Could you check a few things on this model? Use its own coordinates, in mm. Face numbers are marked on the shaded views. A direction names the side the tool comes from. Give positions to 0.01 mm unless a question says otherwise; leave off trailing zeros. Order: outer loops, then holes, each group sorted by start corner. A loop starts at its lowest first (then second) coordinate and runs counter-clockwise, first axis right, second up. Notation, with made-up numbers: M 63.5,68 L 77.5,68 A33 ccw 77.5,102 Z; hole C -13,-21 d2. An arc over 180 degrees is marked long. Answer in a Markdown table with one row per item. Add a question column.
```python
from build123d import *

# Parameters (mm, degrees)
SKETCH_2_R      = 65
SKETCH_2_R_2    = 37.5
EXTRUDE_1_DEPTH = 10
EXTRUDE_2_DEPTH = 50
CHAMFER_1_SIZE  = 10
FILLET_2_R      = 1


with BuildPart() as part:
    # 草圖2 → 填料-伸長1 (new body)
    with BuildSketch(Plane(origin=(0, 0, 0), x_dir=(1, 0, 0), z_dir=(0, 1, 0))):
        with Locations(Location((0, 0, 0), (0, 0, 270))):
            Circle(SKETCH_2_R)
        with Locations(Location((0, 0, 0), (0, 0, 270))):
            Circle(SKETCH_2_R_2, mode=Mode.SUBTRACT)
    extrude(amount=EXTRUDE_1_DEPTH)

    # 草圖3 → 填料-伸長2 (add)
    with BuildSketch(Plane(origin=(0, 10, 0), x_dir=(1, 0, 0), z_dir=(0, 1, 0))):
        with BuildLine():
            Line((-32.475952642, -18.75), (-41.13620668, -23.75))
            ThreePointArc((-41.13620668, -23.75), (0, 47.5), (41.13620668, -23.75))
            Line((41.13620668, -23.75), (32.475952642, -18.75))
            ThreePointArc((32.475952642, -18.75), (0, 37.5), (-32.475952642, -18.75))
        make_face()
    extrude(amount=EXTRUDE_2_DEPTH)

    # 導角1
    # the kernel refuses this chamfer: 10 mm, written as the material it takes off along each edge
    with BuildSketch(Plane(origin=(32.475952642, 10, 18.75), x_dir=(0.35352025121745984, 0, -0.935426871529327), z_dir=(0, 1, 0))) as chamfer_1_piece_1:
        with BuildLine():
            Line((12.116693809, 0), (-CHAMFER_1_SIZE * 0.161555917458, -CHAMFER_1_SIZE * 0.986863559736))
            Line((-CHAMFER_1_SIZE * 0.161555917458, -CHAMFER_1_SIZE * 0.986863559736), (0, 0))
            ThreePointArc((0, 0), (6.22343893, -0.492253103), (12.116693809, 0))
        make_face()
    extrude(amount=81.109263918, mode=Mode.SUBTRACT)
    with BuildSketch(Plane(origin=(-32.475952642, 10, 18.75), x_dir=(-0.3535202512174606, 0, -0.9354268715293267), z_dir=(0, 1, 0))) as chamfer_1_piece_2:
        with BuildLine():
            Line((12.116693809, 0), (-CHAMFER_1_SIZE * 0.161555917458, CHAMFER_1_SIZE * 0.986863559736))
            Line((-CHAMFER_1_SIZE * 0.161555917458, CHAMFER_1_SIZE * 0.986863559736), (0, 0))
            ThreePointArc((0, 0), (6.22343893, 0.492253103), (12.116693809, 0))
        make_face()
    extrude(amount=81.109263918, mode=Mode.SUBTRACT)

    # 圓角2
    fillet_2_edges = [part.edges().sort_by_distance(p)[0] for p in [
        (41.13620668, 35, 23.75),
        (-41.13620668, 35, 23.75),
    ]]
    fillet(fillet_2_edges, radius=FILLET_2_R)


solid = part.part
```
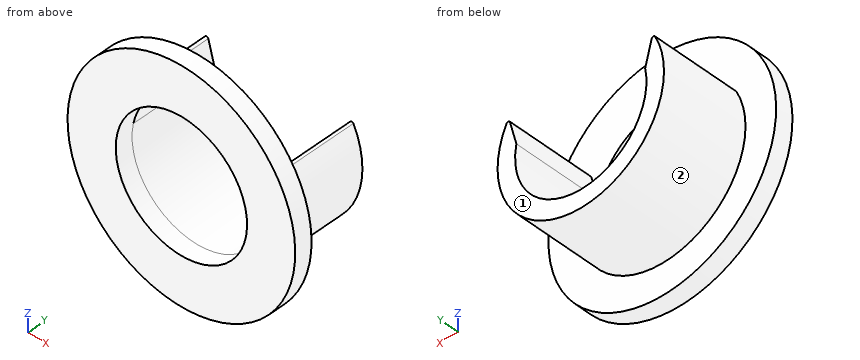
1. Suppose I cut it at A-A on z = 0. List the corners of the cut face in (x, y) for me.
2. Will these pins go through, and if not, where does the flat tip stop? P1, Ø2, axis at y = 41.5, z = -20.5, coming from the -X side; P2, Ø3, axis at x = 6.5, y = 22.5, coming from the +Z side; P3, Ø5, axis at y = 39, z = -39, coming from the -X side.
3. Suppose I cut it at B-B on x = 0. List the corners of the cut face in (y, z) for me.
4. Suppose I cut it at C-C on y = 32. List the corners of the cut face in (x, z) for me, plus the area to 3 significant figures.
5. If I drill on line 1 along X through (y, z) = (5.75, 0); line 2 along X through (y, z) = (25, 0); line 3 along Y through (x, z) = (-40.5, 37), over which ranges is the centre line in solid material (lowest first)? Write a range as [from, to].
6. Suppose I cut it at D-D on z = -40. List the corners of the cut face in (x, y) for me.
7. For the marked faces 1 and 2, which set-ups out of +Z, -Z, +X, -X, +Y, -Y let a thin tool reach every point of the face, with its end or its side?
Findings below:
| question | item | result |
|---|---|---|
| 1 | outline | M -65,0 L -37.5,0 L -37.5,60 L -47.5,60 L -47.5,10 L -65,10 Z; M 37.5,0 L 65,0 L 65,10 L 47.5,10 L 47.5,60 L 37.5,60 Z |
| 2 | P1 | x = -43.31 |
| 2 | P2 | z = -36.64 |
| 2 | P3 | x = -30.4 |
| 3 | outline | M 0,-65 L 10,-65 L 10,-47.5 L 60,-47.5 L 60,-37.5 L 0,-37.5 Z; M 0,37.5 L 10,37.5 L 10,65 L 0,65 Z |
| 4 | outline | M -42.34,21.52 A47.5 ccw long 42.34,21.52 A1 ccw 40.49,21.33 L 36.76,7.42 A37.5 cw long -36.76,7.42 L -40.49,21.33 A1 ccw Z |
| 4 | area | 1,670 mm2 |
| 5 | line 1 | [-65, -37.5], [37.5, 65] |
| 5 | line 2 | [-47.5, -37.5], [37.5, 47.5] |
| 5 | line 3 | [0, 10] |
| 6 | outline | M -51.23,0 L 51.23,0 L 51.23,10 L 25.62,10 L 25.62,60 L -25.62,60 L -25.62,10 L -51.23,10 Z |
| 7 | face 1 | +Z, -Z, +X, -X, +Y |
| 7 | face 2 | +Y |
